Geometry check sheet. Reference: the model listing, model coordinates, mm. Give positions to 0.01 mm unless a question says otherwise; leave off trailing zeros. Write each loop counter-clockwise with the first axis right and the second up, starting at its lowest first coordinate (ties: lowest second). Pieces come first, ordered by that corner, then holes. Notation, with made-up numbers: M -11.5,80 L 8.5,80 A26 ccw 8.5,114 Z; hole C 10.5,48 d3. An arc over 180 degrees is marked long. One line per item, written item: value. Start each with the question number.
1. Cross-section at A-A on x = -27. Record the cut outline in (y, z).
2. Gauge pin test, flat end, axial feed: pin 1 (8 mm diameter, centred on x = -33.5, z = -6.5, fed in from +Y). Record the tip position at first contact, or that the pin passes through.
3. Cross-section at C-C on x = 16. Record the cut outline in (y, z) (3 decimals).
4. Cross-section at B-B on z = -38.5. Record the cut outline in (x, y), then the cut area to 3 significant figures.
5. Scan line: line 1 (Y direction, x = -22, z = -34). Record every from-to range of solid material in increasing order.
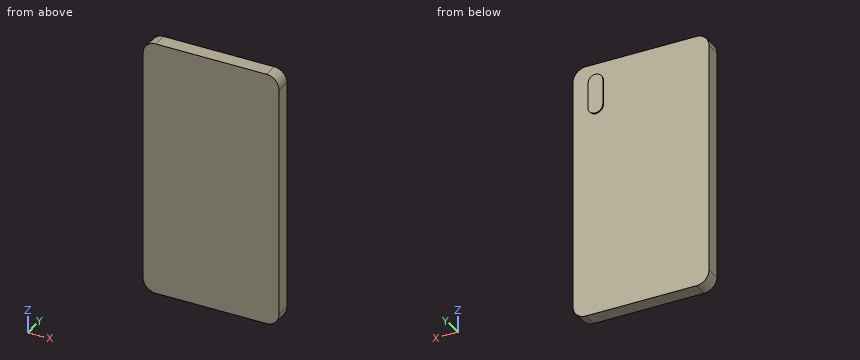
from build123d import *

# Parameters (mm, degrees)
F2_DEPTH = 7.366
F3_W     = 7.4584446847
F3_H     = 12.3723968863
F4_DEPTH = 0.635
F6_DEPTH = 0.635
F7_R     = 1.3168928059
F8_DEPTH = 1.27


with BuildPart() as f2:
    # F1 (on face) → F2 (new body)
    with BuildSketch(Plane.XZ):
        with BuildLine():
            ThreePointArc((25.7346183062, 53.1512381673), (23.8747463667, 57.6413662278), (19.3846183062, 59.5012381673))
            Line((19.3846183062, 59.5012381673), (-36.008353734, 59.5012381673))
            ThreePointArc((-36.008353734, 59.5012381673), (-40.4984817946, 57.6413662278), (-42.358353734, 53.1512381673))
            Line((-42.358353734, 53.1512381673), (-42.358353734, -62.0809899807))
            ThreePointArc((-42.358353734, -62.0809899807), (-40.4984817946, -66.5711180412), (-36.008353734, -68.4309899807))
            Line((-36.008353734, -68.4309899807), (19.3846183062, -68.4309899807))
            ThreePointArc((19.3846183062, -68.4309899807), (23.8747463667, -66.5711180412), (25.7346183062, -62.0809899807))
            Line((25.7346183062, -62.0809899807), (25.7346183062, 53.1512381673))
        make_face()
    extrude(amount=F2_DEPTH)

    # F3 (on face) → F4 (join)
    with BuildSketch(Plane(origin=(0, 0, 0), x_dir=(-1, 0, 0), z_dir=(0, 1, 0))):
        with Locations((-14.2369214445, 43.9156256616)):
            Rectangle(F3_W, F3_H)
    extrude(amount=F4_DEPTH)

    # F5 (on face) → F6 (join)
    with BuildSketch(Plane(origin=(0, 0, 0), x_dir=(-1, 0, 0), z_dir=(0, 1, 0))):
        with BuildLine():
            ThreePointArc((-17.9661437869, 37.7294272184), (-14.2369214445, 34.0002048761), (-10.5076991022, 37.7294272184))
            Line((-10.5076991022, 37.7294272184), (-17.9661437869, 37.7294272184))
        make_face()
        with BuildLine():
            Line((-17.9661437869, 50.1018241048), (-10.5076991022, 50.1018241048))
            ThreePointArc((-10.5076991022, 50.1018241048), (-14.2369214445, 53.8310464472), (-17.9661437869, 50.1018241048))
        make_face()
    extrude(amount=F6_DEPTH)

    # F7 (on face) → F8 (join)
    with BuildSketch(Plane(origin=(0, 0, 0), x_dir=(-1, 0, 0), z_dir=(0, 1, 0))):
        with BuildLine():
            ThreePointArc((-19.3846183062, 59.5012381673), (-23.8747463667, 57.6413662278), (-25.7346183062, 53.1512381673))
            Line((-25.7346183062, 53.1512381673), (-25.7346183062, -62.0809899807))
            ThreePointArc((-25.7346183062, -62.0809899807), (-23.8747463667, -66.5711180412), (-19.3846183062, -68.4309899807))
            Line((-19.3846183062, -68.4309899807), (36.008353734, -68.4309899807))
            ThreePointArc((36.008353734, -68.4309899807), (40.4984817946, -66.5711180412), (42.358353734, -62.0809899807))
            Line((42.358353734, -62.0809899807), (42.358353734, 53.1512381673))
            ThreePointArc((42.358353734, 53.1512381673), (40.4984817946, 57.6413662278), (36.008353734, 59.5012381673))
            Line((36.008353734, 59.5012381673), (-19.3846183062, 59.5012381673))
        make_face()
        with BuildLine():
            Line((-10.5076991022, 50.1018241048), (-10.5076991022, 37.7294272184))
            ThreePointArc((-10.5076991022, 37.7294272184), (-14.2369214445, 34.0002048761), (-17.9661437869, 37.7294272184))
            Line((-17.9661437869, 37.7294272184), (-17.9661437869, 50.1018241048))
            ThreePointArc((-17.9661437869, 50.1018241048), (-14.2369214445, 53.8310464472), (-10.5076991022, 50.1018241048))
        make_face(mode=Mode.SUBTRACT)
        with Locations((-6.3106212765, 47.3092123866)):
            Circle(F7_R, mode=Mode.SUBTRACT)
        with Locations((-6.3106212765, 47.3092123866)):
            Circle(F7_R)
    extrude(amount=-F8_DEPTH)


solid = f2.part
Report:
1. outline: M -7.37,-68.43 L 0,-68.43 L 0,59.5 L -7.37,59.5 Z
2. pin 1: stops at y = 0
3. outline: M -7.366,-68.431 L 0,-68.431 L 0,34.443 L 0.635,34.443 L 0.635,53.388 L 0,53.388 L 0,59.501 L -7.366,59.501 Z
4. outline: M -42.36,-7.37 L 25.73,-7.37 L 25.73,0 L -42.36,0 Z
4. area: 502 mm^2
5. line 1: y = -7.37 to 0
